Could you check a few things on this model? Use its own coordinates, in mm. A direction names the side the tool comes from. Round coordinates to 2 decimals unless told otherwise and drop trailing zeros. Loops run counter-clockwise (first coordinate to the right, second up) from the corner with the lowest first, then second, coordinate; pieces in that order, holes last. Notation, with made-up numbers: (69, 86.25) -> (104, 86.25) arc R30 cw to (104, 119.25) -> close; hole circle Ø10 at (8.25, 80.25). An arc over 180 degrees is marked (long way). One line per item, written item: value.
from build123d import *

# Parameters (mm, degrees)
ESQUISSE1_W             = 27
ESQUISSE1_H             = 27
BOSS_EXTRU_1_DEPTH      = 15
ESQUISSE2_W             = 23
ESQUISSE2_H             = 10
ENL_V_MAT_EXTRU_1_DEPTH = 13
ESQUISSE3_W             = 5
ESQUISSE3_H             = 10
BOSS_EXTRU_2_DEPTH      = 2.2
ESQUISSE4_R             = 0.8
ENL_V_MAT_EXTRU_2_DEPTH = 22.934903693
ENL_V_MAT_EXTRU_3_REACH = 34.129
ESQUISSE5_W             = 10
ESQUISSE5_H             = 11
ENL_V_MAT_EXTRU_4_REACH = 25.098
ESQUISSE6_W             = 2
ESQUISSE6_H             = 10
ESQUISSE7_R             = 1.1
ENL_V_MAT_EXTRU_5_DEPTH = 25.279621084
ENL_V_MAT_EXTRU_6_DEPTH = 12.5
CONG_1_R                = 6
CONG_1_R_2              = 2


with BuildPart() as part:
    # Esquisse1 → Boss.-Extru.1 (new body)
    with BuildSketch(Plane(origin=(0, 0, 0), x_dir=(1, 0, 0), z_dir=(0, 1, 0))):
        Rectangle(ESQUISSE1_W, ESQUISSE1_H)
    extrude(amount=BOSS_EXTRU_1_DEPTH)

    # Esquisse2 → Enlèv. mat.-Extru.1 (cut)
    with BuildSketch(Plane(origin=(0, 15, 0), x_dir=(1, 0, 0), z_dir=(0, 1, 0))):
        Rectangle(ESQUISSE2_W, ESQUISSE2_H)
    extrude(amount=-ENL_V_MAT_EXTRU_1_DEPTH, mode=Mode.SUBTRACT)

    # Esquisse3 → Boss.-Extru.2 (add)
    with BuildSketch(Plane(origin=(0, 2, 0), x_dir=(1, 0, 0), z_dir=(0, 1, 0))):
        with Locations((9, 0)):
            Rectangle(ESQUISSE3_W, ESQUISSE3_H)
    extrude(amount=BOSS_EXTRU_2_DEPTH)

    # Esquisse4 → Enlèv. mat.-Extru.2 (cut, through all)
    with BuildSketch(Plane(origin=(0, 4.2, 0), x_dir=(1, 0, 0), z_dir=(0, 1, 0))):
        with Locations(Location((9, 0, 0), (0, 0, 270))):
            Circle(ESQUISSE4_R)
    extrude(amount=-ENL_V_MAT_EXTRU_2_DEPTH, mode=Mode.SUBTRACT)

    # Esquisse5 → Enlèv. mat.-Extru.3 (cut, up to next)
    with BuildSketch(Plane(origin=(-11.5, 0, 0), x_dir=(0, 0, -1), z_dir=(1, 0, 0)), mode=Mode.PRIVATE) as enl_v_mat_extru_3_sk1:
        with Locations((0, 7.5)):
            Rectangle(ESQUISSE5_W, ESQUISSE5_H)
    enl_v_mat_extru_3_tool1 = extrude(enl_v_mat_extru_3_sk1.sketch, amount=-ENL_V_MAT_EXTRU_3_REACH, mode=Mode.PRIVATE) & part.part
    add(enl_v_mat_extru_3_tool1.solids().sort_by_distance((-11.5, 7.5, 0))[0], mode=Mode.SUBTRACT)

    # Esquisse6 → Enlèv. mat.-Extru.4 (cut, up to next)
    with BuildSketch(Plane(origin=(0, 2, 0), x_dir=(1, 0, 0), z_dir=(0, 1, 0)), mode=Mode.PRIVATE) as enl_v_mat_extru_4_sk1:
        with Locations((-12.5, 0)):
            Rectangle(ESQUISSE6_W, ESQUISSE6_H)
    enl_v_mat_extru_4_tool1 = extrude(enl_v_mat_extru_4_sk1.sketch, amount=-ENL_V_MAT_EXTRU_4_REACH, mode=Mode.PRIVATE) & part.part
    add(enl_v_mat_extru_4_tool1.solids().sort_by_distance((-12.5, 2, 0))[0], mode=Mode.SUBTRACT)

    # Esquisse7 → Enlèv. mat.-Extru.5 (cut, through all)
    with BuildSketch(Plane(origin=(0, 15, 0), x_dir=(1, 0, 0), z_dir=(0, 1, 0))):
        with Locations(Location((0, -9.5, 0), (0, 0, 270))):
            Circle(ESQUISSE7_R)
        with Locations(Location((0, 9.5, 0), (0, 0, 270))):
            Circle(ESQUISSE7_R)
    extrude(amount=-ENL_V_MAT_EXTRU_5_DEPTH, mode=Mode.SUBTRACT)

    # Esquisse8 → Enlèv. mat.-Extru.6 (cut)
    with BuildSketch(Plane.XZ):
        Polygon((2.309401077, -9.5), (1.154700538, -7.5), (-1.154700538, -7.5), (-2.309401077, -9.5), (-1.154700538, -11.5), (1.154700538, -11.5), align=None)
        Polygon((2.309401077, 9.5), (1.154700538, 11.5), (-1.154700538, 11.5), (-2.309401077, 9.5), (-1.154700538, 7.5), (1.154700538, 7.5), align=None)
    extrude(amount=-ENL_V_MAT_EXTRU_6_DEPTH, mode=Mode.SUBTRACT)

    # Enlèv. mat.-Extru.7: read off the stored shape, not the designer's step
    # Enlèv. mat.-Extru.7: loft between two sections, ruled curve by curve
    enl_v_mat_extru_7_from = [
        Edge.make_line((2.771281292, 0, -9.5), (1.385640646, 0, -7.1)),
        Edge.make_line((1.385640646, 0, -7.1), (-1.385640646, 0, -7.1)),
        Edge.make_line((-1.385640646, 0, -7.1), (-2.771281292, 0, -9.5)),
        Edge.make_line((-2.771281292, 0, -9.5), (-1.385640646, 0, -11.9)),
        Edge.make_line((-1.385640646, 0, -11.9), (1.385640646, 0, -11.9)),
        Edge.make_line((1.385640646, 0, -11.9), (2.771281292, 0, -9.5)),
    ]
    enl_v_mat_extru_7_to = [
        Edge.make_line((2.309401077, 5.720266503, -9.5), (1.154700538, 5.720266503, -7.5)),
        Edge.make_line((1.154700538, 5.720266503, -7.5), (-1.154700538, 5.720266503, -7.5)),
        Edge.make_line((-1.154700538, 5.720266503, -7.5), (-2.309401077, 5.720266503, -9.5)),
        Edge.make_line((-2.309401077, 5.720266503, -9.5), (-1.154700538, 5.720266503, -11.5)),
        Edge.make_line((-1.154700538, 5.720266503, -11.5), (1.154700538, 5.720266503, -11.5)),
        Edge.make_line((1.154700538, 5.720266503, -11.5), (2.309401077, 5.720266503, -9.5)),
    ]
    enl_v_mat_extru_7 = Solid(Shell([*[Face.make_surface_from_curves(enl_v_mat_extru_7_from[k], enl_v_mat_extru_7_to[k]) for k in range(6)], Face(Wire(enl_v_mat_extru_7_from)), Face(Wire(enl_v_mat_extru_7_to))]))
    add(enl_v_mat_extru_7, mode=Mode.SUBTRACT)

    # Enl_v. mat.-Extru.7 2: loft between two sections, ruled curve by curve
    enl_v_mat_extru_7_2_from = [
        Edge.make_line((2.771281292, 0, 9.5), (1.385640646, 0, 11.9)),
        Edge.make_line((1.385640646, 0, 11.9), (-1.385640646, 0, 11.9)),
        Edge.make_line((-1.385640646, 0, 11.9), (-2.771281292, 0, 9.5)),
        Edge.make_line((-2.771281292, 0, 9.5), (-1.385640646, 0, 7.1)),
        Edge.make_line((-1.385640646, 0, 7.1), (1.385640646, 0, 7.1)),
        Edge.make_line((1.385640646, 0, 7.1), (2.771281292, 0, 9.5)),
    ]
    enl_v_mat_extru_7_2_to = [
        Edge.make_line((2.309401077, 5.720266503, 9.5), (1.154700538, 5.720266503, 11.5)),
        Edge.make_line((1.154700538, 5.720266503, 11.5), (-1.154700538, 5.720266503, 11.5)),
        Edge.make_line((-1.154700538, 5.720266503, 11.5), (-2.309401077, 5.720266503, 9.5)),
        Edge.make_line((-2.309401077, 5.720266503, 9.5), (-1.154700538, 5.720266503, 7.5)),
        Edge.make_line((-1.154700538, 5.720266503, 7.5), (1.154700538, 5.720266503, 7.5)),
        Edge.make_line((1.154700538, 5.720266503, 7.5), (2.309401077, 5.720266503, 9.5)),
    ]
    enl_v_mat_extru_7_2 = Solid(Shell([*[Face.make_surface_from_curves(enl_v_mat_extru_7_2_from[k], enl_v_mat_extru_7_2_to[k]) for k in range(6)], Face(Wire(enl_v_mat_extru_7_2_from)), Face(Wire(enl_v_mat_extru_7_2_to))]))
    add(enl_v_mat_extru_7_2, mode=Mode.SUBTRACT)

    # Congé1
    # the kernel refuses this fillet: 6, 2 mm, written as the material it takes off along each edge
    with BuildSketch(Plane(origin=(13.5, -15, -13.5), x_dir=(-1, 0, 0), z_dir=(0, 1, 0)), Plane(origin=(13.5, -15, 13.5), x_dir=(0, 0, -1), z_dir=(0, 1, 0))) as cong_1_piece_1:
        with BuildLine():
            CenterArc((CONG_1_R, CONG_1_R), CONG_1_R, 180, 90)
            Line((0, CONG_1_R), (0, 0))
            Line((0, 0), (CONG_1_R, 0))
        make_face()
    extrude(amount=45, mode=Mode.SUBTRACT)
    with BuildSketch(Plane(origin=(-13.5, -15, 13.5), x_dir=(0, 0, -1), z_dir=(0, 1, 0)), Plane(origin=(-13.5, -15, -13.5), x_dir=(1, 0, 0), z_dir=(0, 1, 0))) as cong_1_piece_2:
        with BuildLine():
            CenterArc((CONG_1_R, -CONG_1_R), CONG_1_R, 90, 90)
            Line((0, -CONG_1_R), (0, 0))
            Line((0, 0), (CONG_1_R, 0))
        make_face()
    extrude(amount=45, mode=Mode.SUBTRACT)
    with BuildSketch(Plane(origin=(-11.5, 0, -5), x_dir=(1, 0, 0), z_dir=(0, 0, 1))) as cong_1_piece_3:
        with BuildLine():
            CenterArc((CONG_1_R_2, CONG_1_R_2), CONG_1_R_2, 180, 90)
            Line((0, CONG_1_R_2), (0, 0))
            Line((0, 0), (CONG_1_R_2, 0))
        make_face()
    extrude(amount=10, mode=Mode.SUBTRACT)
    # the kernel refuses this fillet: 6, 2 mm, written as the material it takes off along each edge
    with BuildSketch(Plane(origin=(13.5, 0, -7.5), x_dir=(0, 1, 0), z_dir=(0, 0, 1)), Plane(origin=(-7.5, 0, -13.5), x_dir=(0, 1, 0), z_dir=(1, 0, 0)), Plane(origin=(7.5, 0, 13.5), x_dir=(0, 1, 0), z_dir=(-1, 0, 0))) as cong_1_2_piece_1:
        with BuildLine():
            CenterArc((CONG_1_R_2, CONG_1_R_2), CONG_1_R_2, 180, 90)
            Line((0, CONG_1_R_2), (0, 0))
            Line((0, 0), (CONG_1_R_2, 0))
        make_face()
    extrude(amount=15, mode=Mode.SUBTRACT)
    with BuildSketch(Plane(origin=(-13.5, 0, 0), x_dir=(0, 1, 0), z_dir=(0, 0, -1)), Plane(origin=(-13.5, 0, 7.5), x_dir=(0, 1, 0), z_dir=(0, 0, -1))) as cong_1_2_piece_2:
        with BuildLine():
            CenterArc((CONG_1_R_2, CONG_1_R_2), CONG_1_R_2, 180, 90)
            Line((0, CONG_1_R_2), (0, 0))
            Line((0, 0), (CONG_1_R_2, 0))
        make_face()
    extrude(amount=7.5, mode=Mode.SUBTRACT)
    with BuildSketch(Plane(origin=(-7.5, 0, 7.5), x_dir=(0, 0, 1), z_dir=(1, 0, 0))) as cong_1_2_piece_3:
        with BuildLine():
            CenterArc((6 - CONG_1_R_2, -CONG_1_R_2), CONG_1_R_2, 0, 90)
            Line((6 - CONG_1_R_2, 0), (6, 0))
            Line((6, 0), (6, -CONG_1_R_2))
        make_face()
    revolve(axis=Axis((-7.5, 0, 7.5), (0, -1, 0)), revolution_arc=90, mode=Mode.SUBTRACT)
    with BuildSketch(Plane(origin=(-7.5, 0, -7.5), x_dir=(-1, 0, 0), z_dir=(0, 0, 1))) as cong_1_2_piece_4:
        with BuildLine():
            CenterArc((6 - CONG_1_R_2, -CONG_1_R_2), CONG_1_R_2, 0, 90)
            Line((6 - CONG_1_R_2, 0), (6, 0))
            Line((6, 0), (6, -CONG_1_R_2))
        make_face()
    revolve(axis=Axis((-7.5, 0, -7.5), (0, -1, 0)), revolution_arc=90, mode=Mode.SUBTRACT)
    with BuildSketch(Plane(origin=(7.5, 0, 7.5), x_dir=(1, 0, 0), z_dir=(0, 0, -1))) as cong_1_2_piece_5:
        with BuildLine():
            CenterArc((6 - CONG_1_R_2, -CONG_1_R_2), CONG_1_R_2, 0, 90)
            Line((6 - CONG_1_R_2, 0), (6, 0))
            Line((6, 0), (6, -CONG_1_R_2))
        make_face()
    revolve(axis=Axis((7.5, 0, 7.5), (0, -1, 0)), revolution_arc=90, mode=Mode.SUBTRACT)
    with BuildSketch(Plane(origin=(7.5, 0, -7.5), x_dir=(0, 0, -1), z_dir=(-1, 0, 0))) as cong_1_2_piece_6:
        with BuildLine():
            CenterArc((6 - CONG_1_R_2, -CONG_1_R_2), CONG_1_R_2, 0, 90)
            Line((6 - CONG_1_R_2, 0), (6, 0))
            Line((6, 0), (6, -CONG_1_R_2))
        make_face()
    revolve(axis=Axis((7.5, 0, -7.5), (0, -1, 0)), revolution_arc=90, mode=Mode.SUBTRACT)


solid = part.part
(1) If we section it at C-C, the plane z = 4.5: Please give me the cut outline in (x, y), then the cut area to 3 significant figures.
Recorded:
outline: (-13.5, 13) -> (-11.5, 13) -> (-11.5, 15) -> (-13.5, 15) -> close; (-11.5, 2) arc R2 ccw to (-9.5, 0) -> (11.5, 0) arc R2 ccw to (13.5, 2) -> (13.5, 15) -> (11.5, 15) -> (11.5, 4.2) -> (6.5, 4.2) -> (6.5, 2) -> close
area: 89.3 mm²
(2) Thinking about a two-plate mould opening in X: for faces 1 (the face through (-10.93, 0.6, -0.07)), 2 (the face through (1.74, 9.06, -8.51)), 3 (the face through (9.793, 2.129, -0.104)), 4 (the face through (11.789, 8.409, -11.696)), which applies, released by +X, released by -X, zero draft, split by the parting line, or undercut?
Recorded:
face 1: released by -X
face 2: undercut
face 3: undercut
face 4: released by +X
(3) I'm going to push flat-ended pins straight in: pin 1 Ø2 at (x, z) = (0.5, 9.5) entering from -Y; pin 2 Ø1.1 at (y, z) = (3, -1) entering from -X; pin 3 Ø1.5 at (y, z) = (3, -10) entering from -X. Where does each tip first touch, or does it pass through?
Recorded:
pin 1: y = 12.5
pin 2: x = 6.5
pin 3: x = -13.24
(4) For faces 5 (the face through (-12.9, 0.57, 6.27)), 6 (the face through (8, 4.2, 0)), 7 (the face through (-1.74, 9.06, -10.49)), which set-ups out of +Z, -Z, +X, -X, +Y, -Y let a thin tool reach every point of the face, with its end or its side?
Recorded:
face 5: +Z, -Z, -X, -Y
face 6: -X, +Y
face 7: -Y
(5) If I drill on L1, parallel to Z at x = -4.5, y = 9; L2, parallel to Z at x = -0.25, y = 4; L3, parallel to Z at x = -2, y = 9.75, over which ranges is the centre line in solid material (lowest first)?
Recorded:
L1: -13.5 to -5, 5 to 13.5
L2: -13.5 to -11.62, -7.38 to -5, 5 to 7.38, 11.62 to 13.5
L3: -13.5 to -10.04, -8.96 to -5, 5 to 8.96, 10.04 to 13.5
(6) If we section it at D-D, the plane x = -6.75: Please give me the cut outline in (y, z), then the cut area to 3 significant figures.
Recorded:
outline: (0, -11.5) arc R2 ccw to (2, -13.5) -> (15, -13.5) -> (15, -5) -> (2, -5) -> (2, 5) -> (15, 5) -> (15, 13.5) -> (2, 13.5) arc R2 ccw to (0, 11.5) -> close
area: 273 mm²
(7) If we section it at A-A, the plane z = 0: Please give me the cut outline in (x, y).
Recorded:
outline: (-13.5, 13) -> (-11.5, 13) -> (-11.5, 15) -> (-13.5, 15) -> close; (-11.5, 2) arc R2 ccw to (-9.5, 0) -> (8.2, 0) -> (8.2, 4.2) -> (6.5, 4.2) -> (6.5, 2) -> close; (9.8, 0) -> (11.5, 0) arc R2 ccw to (13.5, 2) -> (13.5, 15) -> (11.5, 15) -> (11.5, 4.2) -> (9.8, 4.2) -> close
(8) If we section it at B-B, the plane y = 10.5: Please give me the cut outline in (x, z), then the cut area to 3 significant figures.
Recorded:
outline: (-13.5, -7.5) arc R6 ccw to (-7.5, -13.5) -> (7.5, -13.5) arc R6 ccw to (13.5, -7.5) -> (13.5, 7.5) arc R6 ccw to (7.5, 13.5) -> (-7.5, 13.5) arc R6 ccw to (-13.5, 7.5) -> (-13.5, 5) -> (11.5, 5) -> (11.5, -5) -> (-13.5, -5) -> close; hole (-2.31, -9.5) -> (-1.15, -11.5) -> (1.15, -11.5) -> (2.31, -9.5) -> (1.15, -7.5) -> (-1.15, -7.5) -> close; hole (-2.31, 9.5) -> (-1.15, 7.5) -> (1.15, 7.5) -> (2.31, 9.5) -> (1.15, 11.5) -> (-1.15, 11.5) -> close
area: 420 mm²
